For this review, take the finished solid that the model builds, in its own axes (mm). A direction names the side the tool comes from. Round coordinates to 2 decimals unless told otherwise and drop trailing zeros. Write each loop counter-clockwise with the first axis right and the second up, starting at its lowest first coordinate (ties: lowest second). Pieces come first, ordered by that corner, then holes. Notation, with made-up numbers: (65, 74) -> (92, 74) arc R13 cw to (92, 92) -> close; hole circle Ø3 at (64.25, -30). An arc over 180 degrees is marked (long way). Answer as CSV lines item,"result". Start each with the question number.
Item 1: Take a section at A-A on z = -14.5. Give the boundary of the cut face in (x, y) (3 decimals), then the cut area to 3 significant figures.
Item 2: Wall thickness on probe 1 along Y at (x, z) = (8, 9); probe 2 along Y at (x, z) = (-7, 20.5); probe 3 along X at (y, z) = (-3, 10.5) (3 decimals): over which ranges is each line inside the solid? List them lowest first. Write a range as from..to.
Item 3: Take a section at C-C on x = -5. Give the boundary of the cut face in (y, z) (3 decimals), then the cut area to 3 significant figures.
Item 4: Take a section at B-B on y = -2. Give the boundary of the cut face in (x, z) (3 decimals).
Item 5: Take a section at D-D on y = 38.1. Give the boundary of the cut face in (x, z) (3 decimals), then the cut area to 3 significant figures.
Item 6: Machinability: for faces 4 (the flat face through (-25.4, 39, 18)), 5 (the flat face through (-14, 3.175, -5)), 6 (the cylindrical face through (0.133, 38.868, 34.917)), which of the approach directions +Z, -Z, +X, -X, +Y, -Y give a long, thin tool a straight path to every point of the face, cutting with its end or side? Answer none if there is none.
Item 7: Mouldability with a two-part tool opening along X and no side actions: class faces 1 (the cylindrical face through (-14.31, -12.202, -11.232)), 2 (the flat face through (-12.7, -6, -4)), 3 (the flat face through (25.4, 39, 18)) as +X half, -X half, draft (parallel to the pull), parting line (faces both ways), or undercut.
Item 8: For pin 1 Ø17 at (y, z) = (-1.5, 3) entering from -X; pin 2 Ø6 at (x, y) = (12.5, 28.5) entering from +Z; pin 3 Ø10.5 at (y, z) = (-8, -2) entering from +X (3 decimals); pin 4 Ø2 at (x, y) = (-16, 44.5) entering from +Z, all flat-tipped, find the tip position at first contact; note any pin that passes through.
```python
from build123d import *

# Parameters (mm, degrees)
BOSS_EXTRUDE1_DEPTH = 25.4
SHELL1_T            = -3.175
SKETCH4_R           = 12.7
BOSS_EXTRUDE3_DEPTH = 15.875
BOSS_EXTRUDE4_DEPTH = 15.875
SKETCH6_R           = 12.7
CUT_EXTRUDE2_DEPTH  = 12.7
CUT_EXTRUDE3_START  = 12.7
SKETCH6_2_R         = 12.7
CUT_EXTRUDE3_DEPTH  = 12.7
CUT_EXTRUDE4_REACH  = 96.666
SKETCH7_R           = 3.175
BOSS_EXTRUDE5_REACH = 96.666
CUT_EXTRUDE5_DEPTH  = 12.7
BOSS_EXTRUDE6_DEPTH = 25.4
FILLET2_R           = 12.7


with BuildPart() as part:
    # Sketch2 → Boss-Extrude1 (new, symmetric)
    with BuildSketch(Plane(origin=(0, 0, 0), x_dir=(0, 0, -1), z_dir=(1, 0, 0))):
        with BuildLine():
            Line((0, 0), (0, 76.2))
            ThreePointArc((0, 76.2), (-38.1, 38.1), (0, 0))
        make_face()
    extrude(amount=BOSS_EXTRUDE1_DEPTH, both=True)

    # Shell1
    shell1_openings = [part.faces().sort_by_distance(p)[0] for p in [
        (0, 38.1, 0),
    ]]
    offset(amount=SHELL1_T, openings=shell1_openings)



with BuildPart() as body_2:
    # Sketch4 → Boss-Extrude3 (new, symmetric)
    with BuildSketch(Plane(origin=(0, 0, 0), x_dir=(0, 0, -1), z_dir=(1, 0, 0))):
        with Locations((9.525, -9.525)):
            Circle(SKETCH4_R)
    extrude(amount=BOSS_EXTRUDE3_DEPTH, both=True)


with BuildPart() as part_1:
    add(part.part)

    add(body_2.part)  # Boss-Extrude4 merges body 2
    # Sketch5 → Boss-Extrude4 (add, symmetric)
    with BuildSketch(Plane(origin=(0, 0, 0), x_dir=(0, 0, -1), z_dir=(1, 0, 0))):
        with BuildLine():
            Line((0, 3.175), (0, 0))
            Line((0, 0), (1.124739587, 0))
            ThreePointArc((1.124739587, 0), (5.034871939, 2.354762203), (9.525, 3.175))
            Line((9.525, 3.175), (0, 3.175))
        make_face()
    extrude(amount=BOSS_EXTRUDE4_DEPTH, both=True)

    # Sketch6 → Cut-Extrude2 (cut)
    with BuildSketch(Plane(origin=(0, 0, 0), x_dir=(0, 0, -1), z_dir=(1, 0, 0))):
        with Locations((8.980256121, -8.980256121)):
            Circle(SKETCH6_R)
    extrude(amount=-CUT_EXTRUDE2_DEPTH, mode=Mode.SUBTRACT)

    # Sketch6<2> → Cut-Extrude3 (cut)
    with BuildSketch(Plane(origin=(0, 0, 0), x_dir=(0, 0, -1), z_dir=(1, 0, 0)).offset(CUT_EXTRUDE3_START)):
        with Locations((8.980256121, -8.980256121)):
            Circle(SKETCH6_2_R)
    extrude(amount=-CUT_EXTRUDE3_DEPTH, mode=Mode.SUBTRACT)

    # Cut-Extrude4: up to this face of the body (flat: up to its plane)
    cut_extrude4_end = Plane(part_1.part.faces().sort_by_distance((15.875, -9.258016607, -9.360446087))[0])
    # Sketch7 → Cut-Extrude4 (cut, up to the picked face)
    with BuildSketch(Plane.ZY.offset(15.875), mode=Mode.PRIVATE) as cut_extrude4_sk1:
        with Locations(Location((-9.525, -9.525, 0), (0, 0, 180))):
            Circle(SKETCH7_R)
    cut_extrude4_tool1 = split(extrude(cut_extrude4_sk1.sketch, amount=-CUT_EXTRUDE4_REACH, mode=Mode.PRIVATE), bisect_by=cut_extrude4_end, keep=Keep.BOTH, mode=Mode.PRIVATE)
    add(cut_extrude4_tool1.solids().sort_by(Axis((-15.875, -9.525, -9.525), (1, 0, 0)))[0], mode=Mode.SUBTRACT)

    # Boss-Extrude5: up to this face of the body (flat: up to its plane)
    boss_extrude5_end = Plane(part_1.part.faces().sort_by_distance((-15.875, 2.815789755, -4.7625))[0])
    # Sketch8 → Boss-Extrude5 (add, up to the picked face)
    with BuildSketch(Plane(origin=(15.875, 0, 0), x_dir=(0, 0, -1), z_dir=(1, 0, 0)), mode=Mode.PRIVATE) as boss_extrude5_sk1:
        with BuildLine():
            Line((-27.936104056, 12.192779189), (0.212965315, -18.16074027))
            Line((0.212965315, -18.16074027), (5.034871939, -21.404762203))
            Line((5.034871939, -21.404762203), (1.124739587, 0))
            Line((1.124739587, 0), (0, 3.175))
            ThreePointArc((0, 3.175), (-13.704863106, 5.9762961), (-25.211222013, 13.9308066))
            Line((-25.211222013, 13.9308066), (-27.936104056, 12.192779189))
        make_face()
    boss_extrude5_tool1 = split(extrude(boss_extrude5_sk1.sketch, amount=-BOSS_EXTRUDE5_REACH, mode=Mode.PRIVATE), bisect_by=boss_extrude5_end, keep=Keep.BOTH, mode=Mode.PRIVATE)
    add(boss_extrude5_tool1.solids().sort_by(Axis((15.875, -2.840531, 7.724646), (-1, 0, 0)))[0])

    # Sketch9 → Cut-Extrude5 (cut, symmetric)
    with BuildSketch(Plane(origin=(0, 0, 0), x_dir=(0, 0, -1), z_dir=(1, 0, 0))):
        with BuildLine():
            Line((0, 3.175), (0, 0))
            ThreePointArc((0, 0), (-15.240486985, 3.180985746), (-27.936104056, 12.192779189))
            Line((-27.936104056, 12.192779189), (0.212965315, -18.16074027))
            ThreePointArc((0.212965315, -18.16074027), (21.164671418, -14.605162328), (9.525, 3.175))
            Line((9.525, 3.175), (0, 3.175))
        make_face()
    extrude(amount=CUT_EXTRUDE5_DEPTH, both=True, mode=Mode.SUBTRACT)

    # Sketch11 → Boss-Extrude6 (add, symmetric)
    with BuildSketch(Plane(origin=(0, 0, 0), x_dir=(0, 0, -1), z_dir=(1, 0, 0))):
        Polygon((2.609832197, 76.2), (0, 76.2), (0, 73.025), align=None)
    extrude(amount=BOSS_EXTRUDE6_DEPTH, both=True)

    # Fillet2
    # the kernel refuses this fillet: 12.7 mm, written as the material it adds along each edge
    with BuildSketch(Plane(origin=(-22.225, 38.1, 0), x_dir=(0, 1, 0), z_dir=(0, 0, -1))) as fillet2_piece_1:
        with BuildLine():
            CenterArc((34.925 - FILLET2_R, FILLET2_R), FILLET2_R, 270, 90)
            Line((34.925 - FILLET2_R, 0), (34.925, 0))
            Line((34.925, 0), (34.925, FILLET2_R))
        make_face()
    revolve(axis=Axis((-22.225, 38.1, 0), (1, 0, 0)), revolution_arc=180)
    with BuildSketch(Plane(origin=(22.225, 38.1, 0), x_dir=(0, 1, 0), z_dir=(0, 0, -1))) as fillet2_piece_2:
        with BuildLine():
            CenterArc((34.925 - FILLET2_R, -FILLET2_R), FILLET2_R, 0, 90)
            Line((34.925 - FILLET2_R, 0), (34.925, 0))
            Line((34.925, 0), (34.925, -FILLET2_R))
        make_face()
    revolve(axis=Axis((22.225, 38.1, 0), (1, 0, 0)), revolution_arc=180)


solid = part_1.part
```
Output values:
1,outline,"(-15.875, -21.21) -> (-12.7, -21.21) -> (-12.7, 2.16) -> (-15.875, 2.16) -> close; (12.7, -21.21) -> (15.875, -21.21) -> (15.875, 2.16) -> (12.7, 2.16) -> close"
1,area,"148 mm^2"
2,probe 1,"y = 1.08..4.35, 71.85..75.12"
2,probe 2,"y = 5.99..9.82, 66.38..70.21"
2,probe 3,"x = -15.875..-12.7, 12.7..15.875"
3,outline,"(0, 0) -> (3.175, 0) arc R34.925 cw to (73.025, 0) -> (76.2, -2.61) -> (76.2, 0) arc R38.1 ccw to start"
3,area,"368 mm^2"
4,outline,"(-15.875, -19.756) -> (-12.7, -19.756) -> (-12.7, 14.774) -> (-15.875, 14.774) -> close; (12.7, -19.756) -> (15.875, -19.756) -> (15.875, 14.774) -> (12.7, 14.774) -> close"
5,outline,"(-25.4, 0) -> (-22.225, 0) -> (-22.225, 22.225) arc R12.7 cw to (-9.525, 34.925) -> (9.525, 34.925) arc R12.7 cw to (22.225, 22.225) -> (22.225, 0) -> (25.4, 0) -> (25.4, 38.1) -> (-25.4, 38.1) -> close"
5,area,"452 mm^2"
6,face 4,"+Z, -Z, -X, +Y, -Y"
6,face 5,"-Z, +X, -X"
6,face 6,"-Z"
7,face 1,"draft"
7,face 2,"undercut"
7,face 3,"+X half"
8,pin 1,"stops at x = -25.4"
8,pin 2,"stops at z = 37.52"
8,pin 3,"stops at x = 15.875"
8,pin 4,"stops at z = 37.72"
